from build123d import *

# Parameters (mm, degrees)
BOSS_EXTRUDE1_DEPTH = 5


with BuildPart() as part:
    # Sketch1 → Boss-Extrude1 (new body)
    with BuildSketch(Plane.XY):
        with BuildLine():
            Line((-122.533931464, 0), (0, 0))
            Line((0, 0), (0, 4))
            Line((0, 4), (-5, 4))
            Line((-5, 4), (-5, 8.902615006))
            Line((-5, 8.902615006), (-5, 13.902615006))
            Line((-5, 13.902615006), (-5, 18.32224988))
            Line((-5, 18.32224988), (-22, 18.32224988))
            Line((-22, 18.32224988), (-22, 52.463633889))
            Line((-22, 52.463633889), (-5, 52.463633889))
            Line((-5, 52.463633889), (-5, 70.203021905))
            Line((-5, 70.203021905), (0, 70.203021905))
            Line((0, 70.203021905), (0, 86.350886134))
            Line((0, 86.350886134), (-182.7, 86.350886134))
            Line((-182.7, 86.350886134), (-182.7, 63.94896177))
            Line((-182.7, 63.94896177), (-160.256841342, 63.94896177))
            Line((-160.256841342, 63.94896177), (-130.724497172, 61.709515068))
            ThreePointArc((-130.724497172, 61.709515068), (-126.402059121, 59.039154196), (-123.878576155, 54.629354699))
            Line((-123.878576155, 54.629354699), (-125.011418309, 37.548381087))
            Line((-125.011418309, 37.548381087), (-82.810223158, 37.548381087))
            ThreePointArc((-82.810223158, 37.548381087), (-80.060223158, 34.798381087), (-82.810223158, 32.048381087))
            Line((-82.810223158, 32.048381087), (-125.427965277, 32.048381087))
            Line((-125.427965277, 32.048381087), (-126.301759952, 20.510976937))
            ThreePointArc((-126.301759952, 20.510976937), (-135.219115409, 13.694571486), (-145.410596187, 8.991771131))
            Line((-145.410596187, 8.991771131), (-182.7, 8.991771131))
            Line((-182.7, 8.991771131), (-182.7, 0))
            Line((-182.7, 0), (-122.533931464, 0))
        make_face()
    extrude(amount=BOSS_EXTRUDE1_DEPTH)


solid = part.part
The model under review builds one solid part; all positions refer to its coordinate system, in mm. A direction names the side the tool comes from. Round coordinates to 2 decimals unless told otherwise and drop trailing zeros. Write each loop counter-clockwise with the first axis right and the second up, starting at its lowest first coordinate (ties: lowest second). Pieces come first, ordered by that corner, then holes. Notation, with made-up numbers: M 69.5,-31 L 115.5,-31 A21 cw 115.5,-26 Z; hole C 89,84 d1. An arc over 180 degrees is marked long. Answer as CSV lines item,"result". Start each with the question number.
Q1. Clearance check with a flat-ended pin moving along its axis: P1, Ø2, axis at y = 19, z = 2, coming from the +X side. State where the tip first meets the part, or that it passes through.
Q2. Consider section B-B, the plane z = 2.6. Give the boundary of the cut face in (x, y), then the cut area to 3 significant figures.
Q3. Wall thickness on line 1 along Y through (x, z) = (-170.5, 4.6); line 2 along Y through (x, z) = (-95, 3.35); line 3 along X through (y, z) = (7.5, 2.4): over which ranges is each line inside the solid? List them lowest first.
Q4. Consider section C-C, the plane x = -150.5. Give the boundary of the cut face in (y, z), then the cut area to 3 significant figures.
Q5. Tool access review of faces 4 (the face through (-182.7, 5, 2)), 5 (the face through (-125.86, 26.36, 2.46)), 6 (the face through (-14, 52.464, 2)): name each direction out of +Z, -Z, +X, -X, +Y, -Y from which nothing blocks a thin tool from reaching the whole face with its end or side.
Q6. Consider section D-D, the plane y = 25. Give the boundary of the cut face in (x, z), then the cut area to 3 significant figures.
Q7. The part is to be moulded in two halves that separate along Y. For faces 1 (the face through (-90, 86.351, 2)), 2 (the face through (-93, 0, 2)), 3 (the face through (-22, 35, 2)), say which applies: +Y half, -Y half, draft (parallel to the pull), parting line (faces both ways), or undercut.
Q8. Consider section A-A, the plane x = -122. Give the boundary of the cut face in (y, z), then the cut area to 3 significant figures.
Result set:
1,P1,"stops at x = -5"
2,outline,"M -182.7,0 L 0,0 L 0,4 L -5,4 L -5,18.32 L -22,18.32 L -22,52.46 L -5,52.46 L -5,70.2 L 0,70.2 L 0,86.35 L -182.7,86.35 L -182.7,63.95 L -160.26,63.95 L -130.72,61.71 A10.32 cw -123.88,54.63 L -125.01,37.55 L -82.81,37.55 A2.75 cw -82.81,32.05 L -125.43,32.05 L -126.3,20.51 A51.05 cw -145.41,8.99 L -182.7,8.99 Z"
2,area,"11,600 mm²"
3,line 1,"y = 0 to 8.99, 63.95 to 86.35"
3,line 2,"y = 0 to 32.05, 37.55 to 86.35"
3,line 3,"x = -182.7 to -5"
4,outline,"M 0,0 L 8.99,0 L 8.99,5 L 0,5 Z; M 63.21,0 L 86.35,0 L 86.35,5 L 63.21,5 Z"
4,area,"161 mm²"
5,face 4,"+Z, -Z, -X, +Y, -Y"
5,face 5,"+Z, -Z, -X"
5,face 6,"+Z, -Z, +X"
6,outline,"M -125.96,0 L -22,0 L -22,5 L -125.96,5 Z"
6,area,"520 mm²"
7,face 1,"+Y half"
7,face 2,"-Y half"
7,face 3,"undercut"
8,outline,"M 0,0 L 32.05,0 L 32.05,5 L 0,5 Z; M 37.55,0 L 86.35,0 L 86.35,5 L 37.55,5 Z"
8,area,"404 mm²"
